Part print with two shaded views. Sizes in mm from the minimum x, y, z corner. A direction names the side the tool comes from. Round coordinates to 2 decimals unless told otherwise and drop trailing zeros. Write each loop counter-clockwise with the first axis right and the second up, starting at its lowest first coordinate (ties: lowest second). Pieces come first, ordered by that corner, then holes. Notation, with made-up numbers: (-9.5, 60) -> (17.5, 60) arc R31 ccw to (17.5, 90) -> close; hole circle Ø4 at (7.25, -7.5). An arc over 180 degrees is marked (long way). Answer in a Markdown table with one row per item.
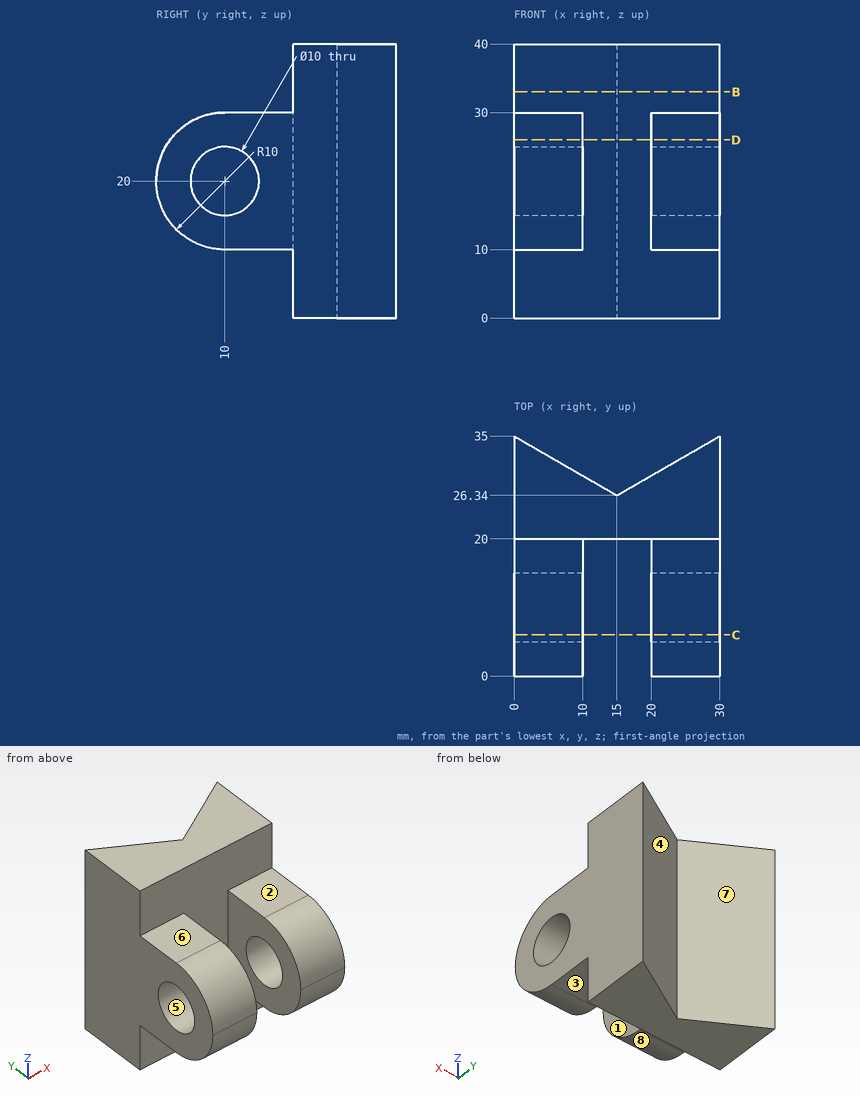
Q1. Saw through at D-D on z = 26. Write the cut outline in (x, y).
A:
| item | result |
|---|---|
| outline | (0, 2) -> (10, 2) -> (10, 20) -> (20, 20) -> (20, 2) -> (30, 2) -> (30, 35) -> (15, 26.34) -> (0, 35) -> close |
Q2. Two-plate mould, pull along Y, no slides. Class the marked faces 5, 6, 7 and 8: released by +Y, released by -Y, zero draft, split by the parting line, or undercut.
A:
| item | result |
|---|---|
| face 5 | undercut |
| face 6 | zero draft |
| face 7 | released by +Y |
| face 8 | released by -Y |
Q3. Saw through at B-B on z = 33. Write the cut outline in (x, y).
A:
| item | result |
|---|---|
| outline | (0, 20) -> (30, 20) -> (30, 35) -> (15, 26.34) -> (0, 35) -> close |
Q4. Which spindle directions (+Z, -Z, +X, -X, +Y, -Y) get a long thin tool onto all of the face, cutting with end or side? Do the marked faces 1, 2, 3 and 4. Say none if no direction does.
A:
| item | result |
|---|---|
| face 1 | +Z, -Z, -Y |
| face 2 | +Z, +X, -X, -Y |
| face 3 | -Z, +X, -X, -Y |
| face 4 | +Z, -Z, +Y |
Q5. Wall check: line 1 (X direction, y = 2, z = 15.5); line 2 (Z direction, x = 24.25, y = 10); line 3 (X direction, y = 27.5, z = 4). Give the ranges that are in metal, low to high. Write a range as [from, to].
A:
| item | result |
|---|---|
| line 1 | [0, 10], [20, 30] |
| line 2 | [10, 15], [25, 30] |
| line 3 | [0, 12.99], [17.01, 30] |
Q6. Drop flat-ended pins along their axis: P1, Ø15, axis at x = 11, z = 29, coming from the -Y side; P2, Ø3, axis at x = 6, y = 14.5, coming from the +Z side; P3, Ø11, axis at x = 3, y = 13, coming from the -Z side. Give the stop position or say it passes through.
A:
| item | result |
|---|---|
| P1 | y = 0.12 |
| P2 | z = 30 |
| P3 | z = 10 |
Q7. Saw through at C-C on y = 6. Write the cut outline in (x, z) (1 decimal).
A:
| item | result |
|---|---|
| outline | (0, 10.8) -> (10, 10.8) -> (10, 17) -> (0, 17) -> close; (0, 23) -> (10, 23) -> (10, 29.2) -> (0, 29.2) -> close; (20, 10.8) -> (30, 10.8) -> (30, 17) -> (20, 17) -> close; (20, 23) -> (30, 23) -> (30, 29.2) -> (20, 29.2) -> close |
